Part model, mm, in its own coordinate system. A direction names the side the tool comes from. Give positions to 0.01 mm unless a question says otherwise; leave off trailing zeros. Order: outer loops, then holes, each group sorted by start corner. A loop starts at its lowest first (then second) coordinate and runs counter-clockwise, first axis right, second up. Notation, with made-up numbers: M 84.25,-29 L 140.25,-29 A19 ccw 140.25,-21 Z; hole C 69.5,6.5 d1. An arc over 180 degrees is marked long. Write each question's results on one line, items separated by ' | '. Start each with the question number.
from build123d import *

# Parameters (mm, degrees)
BOSS_EXTRUDE1_DEPTH     = 10
CUT_EXTRUDE1_DEPTH      = 1
CUT_EXTRUDE1_DEPTH_BACK = 11
SKETCH4_R               = 4.7625
CUT_EXTRUDE2_DEPTH      = 11
SKETCH5_R               = 3.175
CUT_EXTRUDE3_DEPTH      = 11
SKETCH6_R               = 3.175
CUT_EXTRUDE4_DEPTH      = 11
SKETCH7_R               = 3.302
CUT_EXTRUDE5_DEPTH      = 11


with BuildPart() as part:
    # Sketch1 → Boss-Extrude1 (new body)
    with BuildSketch(Plane(origin=(0, 0, 0), x_dir=(1, 0, 0), z_dir=(0, 1, 0))):
        Polygon((0, 279.4), (0, 0), (38.1, 0), (292.1, 0), (361.95, 0), (361.95, 279.4), align=None)
    extrude(amount=BOSS_EXTRUDE1_DEPTH)

    # Sketch2 → Cut-Extrude1 (cut, two sides)
    with BuildSketch(Plane(origin=(0, 10, 0), x_dir=(1, 0, 0), z_dir=(0, 1, 0))) as cut_extrude1_sk:
        with BuildLine():
            Line((350.8375, 270.764), (354.0125, 270.764))
            ThreePointArc((354.0125, 270.764), (358.0765, 266.7), (354.0125, 262.636))
            Line((354.0125, 262.636), (350.8375, 262.636))
            ThreePointArc((350.8375, 262.636), (346.7735, 266.7), (350.8375, 270.764))
        make_face()
        with BuildLine():
            Line((350.8375, 245.364), (354.0125, 245.364))
            ThreePointArc((354.0125, 245.364), (358.0765, 241.3), (354.0125, 237.236))
            Line((354.0125, 237.236), (350.8375, 237.236))
            ThreePointArc((350.8375, 237.236), (346.7735, 241.3), (350.8375, 245.364))
        make_face()
        with BuildLine():
            Line((350.8375, 219.964), (354.0125, 219.964))
            ThreePointArc((354.0125, 219.964), (358.0765, 215.9), (354.0125, 211.836))
            Line((354.0125, 211.836), (350.8375, 211.836))
            ThreePointArc((350.8375, 211.836), (346.7735, 215.9), (350.8375, 219.964))
        make_face()
        with BuildLine():
            Line((350.8375, 194.564), (354.0125, 194.564))
            ThreePointArc((354.0125, 194.564), (358.0765, 190.5), (354.0125, 186.436))
            Line((354.0125, 186.436), (350.8375, 186.436))
            ThreePointArc((350.8375, 186.436), (346.7735, 190.5), (350.8375, 194.564))
        make_face()
        with BuildLine():
            Line((350.8375, 169.164), (354.0125, 169.164))
            ThreePointArc((354.0125, 169.164), (358.0765, 165.1), (354.0125, 161.036))
            Line((354.0125, 161.036), (350.8375, 161.036))
            ThreePointArc((350.8375, 161.036), (346.7735, 165.1), (350.8375, 169.164))
        make_face()
        with BuildLine():
            Line((350.8375, 143.764), (354.0125, 143.764))
            ThreePointArc((354.0125, 143.764), (358.0765, 139.7), (354.0125, 135.636))
            Line((354.0125, 135.636), (350.8375, 135.636))
            ThreePointArc((350.8375, 135.636), (346.7735, 139.7), (350.8375, 143.764))
        make_face()
        with BuildLine():
            Line((350.8375, 118.364), (354.0125, 118.364))
            ThreePointArc((354.0125, 118.364), (358.0765, 114.3), (354.0125, 110.236))
            Line((354.0125, 110.236), (350.8375, 110.236))
            ThreePointArc((350.8375, 110.236), (346.7735, 114.3), (350.8375, 118.364))
        make_face()
        with BuildLine():
            Line((350.8375, 92.964), (354.0125, 92.964))
            ThreePointArc((354.0125, 92.964), (358.0765, 88.9), (354.0125, 84.836))
            Line((354.0125, 84.836), (350.8375, 84.836))
            ThreePointArc((350.8375, 84.836), (346.7735, 88.9), (350.8375, 92.964))
        make_face()
        with BuildLine():
            Line((350.8375, 67.564), (354.0125, 67.564))
            ThreePointArc((354.0125, 67.564), (358.0765, 63.5), (354.0125, 59.436))
            Line((354.0125, 59.436), (350.8375, 59.436))
            ThreePointArc((350.8375, 59.436), (346.7735, 63.5), (350.8375, 67.564))
        make_face()
        with BuildLine():
            Line((350.8375, 42.164), (354.0125, 42.164))
            ThreePointArc((354.0125, 42.164), (358.0765, 38.1), (354.0125, 34.036))
            Line((354.0125, 34.036), (350.8375, 34.036))
            ThreePointArc((350.8375, 34.036), (346.7735, 38.1), (350.8375, 42.164))
        make_face()
        with BuildLine():
            Line((350.8375, 16.764), (354.0125, 16.764))
            ThreePointArc((354.0125, 16.764), (358.0765, 12.7), (354.0125, 8.636))
            Line((354.0125, 8.636), (350.8375, 8.636))
            ThreePointArc((350.8375, 8.636), (346.7735, 12.7), (350.8375, 16.764))
        make_face()
        with BuildLine():
            Line((11.1125, 270.764), (7.9375, 270.764))
            ThreePointArc((7.9375, 270.764), (3.8735, 266.7), (7.9375, 262.636))
            Line((7.9375, 262.636), (11.1125, 262.636))
            ThreePointArc((11.1125, 262.636), (15.1765, 266.7), (11.1125, 270.764))
        make_face()
        with BuildLine():
            Line((11.1125, 16.764), (7.9375, 16.764))
            ThreePointArc((7.9375, 16.764), (3.8735, 12.7), (7.9375, 8.636))
            Line((7.9375, 8.636), (11.1125, 8.636))
            ThreePointArc((11.1125, 8.636), (15.1765, 12.7), (11.1125, 16.764))
        make_face()
        with BuildLine():
            Line((11.1125, 42.164), (7.9375, 42.164))
            ThreePointArc((7.9375, 42.164), (3.8735, 38.1), (7.9375, 34.036))
            Line((7.9375, 34.036), (11.1125, 34.036))
            ThreePointArc((11.1125, 34.036), (15.1765, 38.1), (11.1125, 42.164))
        make_face()
        with BuildLine():
            Line((11.1125, 67.564), (7.9375, 67.564))
            ThreePointArc((7.9375, 67.564), (3.8735, 63.5), (7.9375, 59.436))
            Line((7.9375, 59.436), (11.1125, 59.436))
            ThreePointArc((11.1125, 59.436), (15.1765, 63.5), (11.1125, 67.564))
        make_face()
        with BuildLine():
            Line((11.1125, 92.964), (7.9375, 92.964))
            ThreePointArc((7.9375, 92.964), (3.8735, 88.9), (7.9375, 84.836))
            Line((7.9375, 84.836), (11.1125, 84.836))
            ThreePointArc((11.1125, 84.836), (15.1765, 88.9), (11.1125, 92.964))
        make_face()
        with BuildLine():
            Line((11.1125, 118.364), (7.9375, 118.364))
            ThreePointArc((7.9375, 118.364), (3.8735, 114.3), (7.9375, 110.236))
            Line((7.9375, 110.236), (11.1125, 110.236))
            ThreePointArc((11.1125, 110.236), (15.1765, 114.3), (11.1125, 118.364))
        make_face()
        with BuildLine():
            Line((11.1125, 143.764), (7.9375, 143.764))
            ThreePointArc((7.9375, 143.764), (3.8735, 139.7), (7.9375, 135.636))
            Line((7.9375, 135.636), (11.1125, 135.636))
            ThreePointArc((11.1125, 135.636), (15.1765, 139.7), (11.1125, 143.764))
        make_face()
        with BuildLine():
            Line((11.1125, 169.164), (7.9375, 169.164))
            ThreePointArc((7.9375, 169.164), (3.8735, 165.1), (7.9375, 161.036))
            Line((7.9375, 161.036), (11.1125, 161.036))
            ThreePointArc((11.1125, 161.036), (15.1765, 165.1), (11.1125, 169.164))
        make_face()
        with BuildLine():
            Line((11.1125, 194.564), (7.9375, 194.564))
            ThreePointArc((7.9375, 194.564), (3.8735, 190.5), (7.9375, 186.436))
            Line((7.9375, 186.436), (11.1125, 186.436))
            ThreePointArc((11.1125, 186.436), (15.1765, 190.5), (11.1125, 194.564))
        make_face()
        with BuildLine():
            Line((11.1125, 219.964), (7.9375, 219.964))
            ThreePointArc((7.9375, 219.964), (3.8735, 215.9), (7.9375, 211.836))
            Line((7.9375, 211.836), (11.1125, 211.836))
            ThreePointArc((11.1125, 211.836), (15.1765, 215.9), (11.1125, 219.964))
        make_face()
        with BuildLine():
            Line((11.1125, 245.364), (7.9375, 245.364))
            ThreePointArc((7.9375, 245.364), (3.8735, 241.3), (7.9375, 237.236))
            Line((7.9375, 237.236), (11.1125, 237.236))
            ThreePointArc((11.1125, 237.236), (15.1765, 241.3), (11.1125, 245.364))
        make_face()
    extrude(amount=CUT_EXTRUDE1_DEPTH, mode=Mode.SUBTRACT)
    extrude(cut_extrude1_sk.sketch, amount=-CUT_EXTRUDE1_DEPTH_BACK, mode=Mode.SUBTRACT)

    # Sketch4 → Cut-Extrude2 (cut, through all)
    with BuildSketch(Plane.XZ):
        with Locations((277.8125, -266.7)):
            Circle(SKETCH4_R)
        with Locations((277.8125, -146.05)):
            Circle(SKETCH4_R)
    extrude(amount=-CUT_EXTRUDE2_DEPTH, mode=Mode.SUBTRACT)

    # Sketch5 → Cut-Extrude3 (cut, through all)
    with BuildSketch(Plane.XZ):
        with Locations((257.175, -266.944116923)):
            Circle(SKETCH5_R)
        with Locations((273.05, -222.494116923)):
            Circle(SKETCH5_R)
        with Locations((241.3, -222.494116923)):
            Circle(SKETCH5_R)
    extrude(amount=-CUT_EXTRUDE3_DEPTH, mode=Mode.SUBTRACT)

    # Sketch6 → Cut-Extrude4 (cut, through all)
    with BuildSketch(Plane.XZ):
        with Locations((109.696959753, -228.6)):
            Circle(SKETCH6_R)
        with Locations((109.696959753, -177.8)):
            Circle(SKETCH6_R)
        with Locations((109.696959753, -123.825)):
            Circle(SKETCH6_R)
        with Locations((109.696959753, -73.025)):
            Circle(SKETCH6_R)
        with Locations((160.496959753, -228.6)):
            Circle(SKETCH6_R)
        with Locations((160.496959753, -177.8)):
            Circle(SKETCH6_R)
        with Locations((160.496959753, -123.825)):
            Circle(SKETCH6_R)
        with Locations((160.496959753, -73.025)):
            Circle(SKETCH6_R)
    extrude(amount=-CUT_EXTRUDE4_DEPTH, mode=Mode.SUBTRACT)

    # Sketch7 → Cut-Extrude5 (cut, through all)
    with BuildSketch(Plane.XZ):
        with Locations((25.4, -266.7)):
            Circle(SKETCH7_R)
        with Locations((336.55, -266.7)):
            Circle(SKETCH7_R)
        with Locations((336.55, -12.7)):
            Circle(SKETCH7_R)
        with Locations((25.4, -12.7)):
            Circle(SKETCH7_R)
    extrude(amount=-CUT_EXTRUDE5_DEPTH, mode=Mode.SUBTRACT)


solid = part.part
(1) Tool access for faces 5 (the cylindrical face through (358.076, 5.07, -215.989)), 6 (the flat face through (178, 0, -142)): list every direction of +Z, -Z, +X, -X, +Y, -Y with a clear straight run to the whole face (end or side of a thin tool).
(2) Saw through at A-A on z = -165.1. Give the cut face in (x, y), plus the area to 3 significant figures.
(3) Drop a flat-ended pin along its axis: P1, Ø5, axis at x = 109.7, z = -228.6, coming from the -Y side. Give the stop position or say it passes through.
(4) Pull direction Z, two halves, no side cores. Call faces 1 (the cylindrical face through (358.076, 5.07, -63.589)), 2 (the flat face through (184, 5, -279.4)), 3 (the cylindrical face through (3.874, 5.07, -38.189)), 4 (the flat face through (178, 10, -142)): +Z half, -Z half, draft (parallel to the pull), parting line (faces both ways), or undercut.
(5) Probe L1, parallel to Z at x = 26, y = 7.25; L2, parallel to X at y = 7.25, z = -177.8; L3, parallel to X at y = 3.25, z = -63. List the from-to ranges inside material, lowest first.
(6) Saw through at B-B on y = 6.75. Give the number of separate pieces and of enclosed holes in the cut face, plus the area to 3 significant figures.
Taken from the geometry:
1) face 5: +Y, -Y | face 6: +Z, -Z, +X, -X, -Y
2) outline: M 0,0 L 3.87,0 L 3.87,10 L 0,10 Z; M 15.18,0 L 346.77,0 L 346.77,10 L 15.18,10 Z; M 358.08,0 L 361.95,0 L 361.95,10 L 358.08,10 Z | area: 3,390 mm²
3) P1: passes through
4) face 1: undercut | face 2: -Z half | face 3: undercut | face 4: draft
5) L1: z = -279.4 to -269.95, -263.45 to -15.95, -9.45 to 0 | L2: x = 0 to 106.52, 112.87 to 157.32, 163.67 to 361.95 | L3: x = 0 to 3.9, 15.15 to 346.8, 358.05 to 361.95
6) separate pieces: 1 | enclosed holes: 39 | area: 98,800 mm²
